from build123d import *

# Parameters (mm, degrees)
SKETCH1_W           = 41.2
SKETCH1_H           = 31.2
BOSS_EXTRUDE1_DEPTH = 3
SKETCH2_W           = 25.1
SKETCH2_H           = 31.2
BOSS_EXTRUDE2_DEPTH = 3.7
SKETCH3_R           = 2
CUT_EXTRUDE1_DEPTH  = 3
CUT_EXTRUDE2_REACH  = 28.695
CHAMFER1_SIZE       = 0.5


with BuildPart() as part:
    # Sketch1 → Boss-Extrude1 (new body)
    with BuildSketch(Plane(origin=(0, 0, 0), x_dir=(1, 0, 0), z_dir=(0, 1, 0))):
        Rectangle(SKETCH1_W, SKETCH1_H)
    extrude(amount=BOSS_EXTRUDE1_DEPTH)

    # Sketch2 → Boss-Extrude2 (add)
    with BuildSketch(Plane(origin=(0, 3, 0), x_dir=(1, 0, 0), z_dir=(0, 1, 0))):
        Rectangle(SKETCH2_W, SKETCH2_H)
    extrude(amount=BOSS_EXTRUDE2_DEPTH)

    # Sketch3 → Cut-Extrude1 (cut)
    with BuildSketch(Plane(origin=(0, 3, 0), x_dir=(1, 0, 0), z_dir=(0, 1, 0))):
        with Locations(Location((16.6, -11.6, 0), (0, 0, 270))):
            Circle(SKETCH3_R)
        with Locations(Location((-16.6, -11.6, 0), (0, 0, 270))):
            Circle(SKETCH3_R)
        with Locations(Location((16.6, 11.6, 0), (0, 0, 270))):
            Circle(SKETCH3_R)
        with Locations(Location((-16.6, 11.6, 0), (0, 0, 270))):
            Circle(SKETCH3_R)
    extrude(amount=-CUT_EXTRUDE1_DEPTH, mode=Mode.SUBTRACT)

    # Cut-Extrude2: up to this face of the body (flat: up to its plane)
    cut_extrude2_end = Plane(part.part.faces().sort_by_distance((0, 6.7, 0))[0])
    # Sketch4 → Cut-Extrude2 (cut, up to the picked face)
    with BuildSketch(Plane.XZ, mode=Mode.PRIVATE) as cut_extrude2_sk1:
        Polygon((-7.5, -15.6), (7.5, -15.6), (7.5, -7.6), (12.6, -7.6), (12.6, 7.6), (-12.6, 7.6), (-12.6, -7.6), (-7.5, -7.6), align=None)
    cut_extrude2_tool1 = split(extrude(cut_extrude2_sk1.sketch, amount=-CUT_EXTRUDE2_REACH, mode=Mode.PRIVATE), bisect_by=cut_extrude2_end, keep=Keep.BOTH, mode=Mode.PRIVATE)
    add(cut_extrude2_tool1.solids().sort_by(Axis((0, 0, -2.767176), (0, 1, 0)))[0], mode=Mode.SUBTRACT)

    # Chamfer1
    chamfer1_edges = [part.edges().sort_by_distance(p)[0] for p in [
        (16.6, 0, -13.6),
        (-16.6, 0, 9.6),
        (-16.6, 0, -13.6),
        (16.6, 0, 9.6),
    ]]
    chamfer(chamfer1_edges, length=CHAMFER1_SIZE)


solid = part.part
Geometry: final body of the model. Coordinates: model frame, mm. A direction names the side the tool comes from. Give positions to 0.01 mm unless a question says otherwise; leave off trailing zeros. Write each loop counter-clockwise with the first axis right and the second up, starting at its lowest first coordinate (ties: lowest second). Pieces come first, ordered by that corner, then holes. Notation, with made-up numbers: M 59,-19.75 L 87,-19.75 A13 cw 87,5.25 Z; hole C 68,80 d8. An arc over 180 degrees is marked long. Answer in a Markdown table with one row per item. Add a question column.
(1) Reachability of faces 1 (the flat face through (7.5, 3, -12)), 2 (the flat face through (0, 3, 7.6)), 3 (the flat face through (-12.55, 5, -12)) from +Z, -Z, +X, -X, +Y, -Y: full face, straight path, thin tool, end or side. Return the list, or none.
(2) Ray query, line 1 (X direction, y = 1.3, z = 11.6); line 2 (X direction, y = 1, z = -11.6); line 3 (X direction, y = 2.5, z = 0.5). Return the intervals inside material, ascending.
(3) First-contact query: pin 1 (6.5 mm diameter, centred on x = 16.6, z = -11.6, fed in from -Y); pin 2 (4 mm diameter, centred on y = 5.5, z = -11.5, fed in from -X); pin 3 (6.5 mm diameter, centred on x = 16.6, z = 11.6, fed in from +Y); pin 4 (3.5 mm diameter, centred on x = -3, y = 2, fed in from -Z). Flat tips, straight axial feed; report the tip coordinate or a pass-through.
(4) Section B-B on y = 5.75. Return loops of the section in (x, z).
(5) Section D-D on z = -11.6. Return loops of the section in (x, y).
(6) Section C-C on x = 16.6. Return loops of the section in (y, z), and give its area (3 significant figures).
(7) Mould query, pull axis X, two halves, no side actions, for faces 4 (the flat face through (-20.6, 1, 0)), 5 (the flat face through (12.55, 5, 12)), 6 (the cylindrical face through (-14.914, 1.768, -10.525)). Classes: +X half, -X half, draft (parallel to the pull), parting line (faces both ways), or undercut.
(8) Section A-A on z = 11.6. Return loops of the section in (x, y).
Result set:
| question | item | result |
|---|---|---|
| 1 | face 1 | -Z, +Y, -Y |
| 1 | face 2 | +Y, -Y |
| 1 | face 3 | +Z, -Z, -X, +Y |
| 2 | line 1 | x = -20.6 to -18.6, -14.6 to 14.6, 18.6 to 20.6 |
| 2 | line 2 | x = -20.6 to -18.6, -14.6 to -7.5, 7.5 to 14.6, 18.6 to 20.6 |
| 2 | line 3 | x = -20.6 to -12.6, 12.6 to 20.6 |
| 3 | pin 1 | stops at y = 0 |
| 3 | pin 2 | stops at x = -12.55 |
| 3 | pin 3 | stops at y = 3 |
| 3 | pin 4 | stops at z = 7.6 |
| 4 | outline | M -12.55,-15.6 L -7.5,-15.6 L -7.5,-7.6 L -12.55,-7.6 Z; M -12.55,7.6 L 12.55,7.6 L 12.55,15.6 L -12.55,15.6 Z; M 7.5,-15.6 L 12.55,-15.6 L 12.55,-7.6 L 7.5,-7.6 Z |
| 5 | outline | M -20.6,0 L -19.1,0 L -18.6,0.5 L -18.6,3 L -20.6,3 Z; M -14.6,0.5 L -14.1,0 L -7.5,0 L -7.5,6.7 L -12.55,6.7 L -12.55,3 L -14.6,3 Z; M 7.5,0 L 14.1,0 L 14.6,0.5 L 14.6,3 L 12.55,3 L 12.55,6.7 L 7.5,6.7 Z; M 18.6,0.5 L 19.1,0 L 20.6,0 L 20.6,3 L 18.6,3 Z |
| 6 | outline | M 0,-15.6 L 3,-15.6 L 3,-13.6 L 0.5,-13.6 L 0,-14.1 Z; M 0,-9.1 L 0.5,-9.6 L 3,-9.6 L 3,9.6 L 0.5,9.6 L 0,9.1 Z; M 0,14.1 L 0.5,13.6 L 3,13.6 L 3,15.6 L 0,15.6 Z |
| 6 | area | 69.1 mm^2 |
| 7 | face 4 | -X half |
| 7 | face 5 | +X half |
| 7 | face 6 | undercut |
| 8 | outline | M -20.6,0 L -19.1,0 L -18.6,0.5 L -18.6,3 L -20.6,3 Z; M -14.6,0.5 L -14.1,0 L 14.1,0 L 14.6,0.5 L 14.6,3 L 12.55,3 L 12.55,6.7 L -12.55,6.7 L -12.55,3 L -14.6,3 Z; M 18.6,0.5 L 19.1,0 L 20.6,0 L 20.6,3 L 18.6,3 Z |
